Source: three-view drawing plus pictorial views. Frame: mm from the lowest corner of the part. A direction names the side the tool comes from. Give positions to 0.01 mm unless a question says otherwise; leave off trailing zeros. Loops run counter-clockwise (first coordinate to the right, second up) from the corner with the lowest first, then second, coordinate; pieces in that order, holes last. Notation, with made-up numbers: (-25.75, 68) -> (20.25, 68) arc R38 ccw to (20.25, 106) -> close; hole circle Ø7 at (18, 7). An arc over 180 degrees is marked (long way). Answer as a JSON object with one key per item and string values. Group by question number.
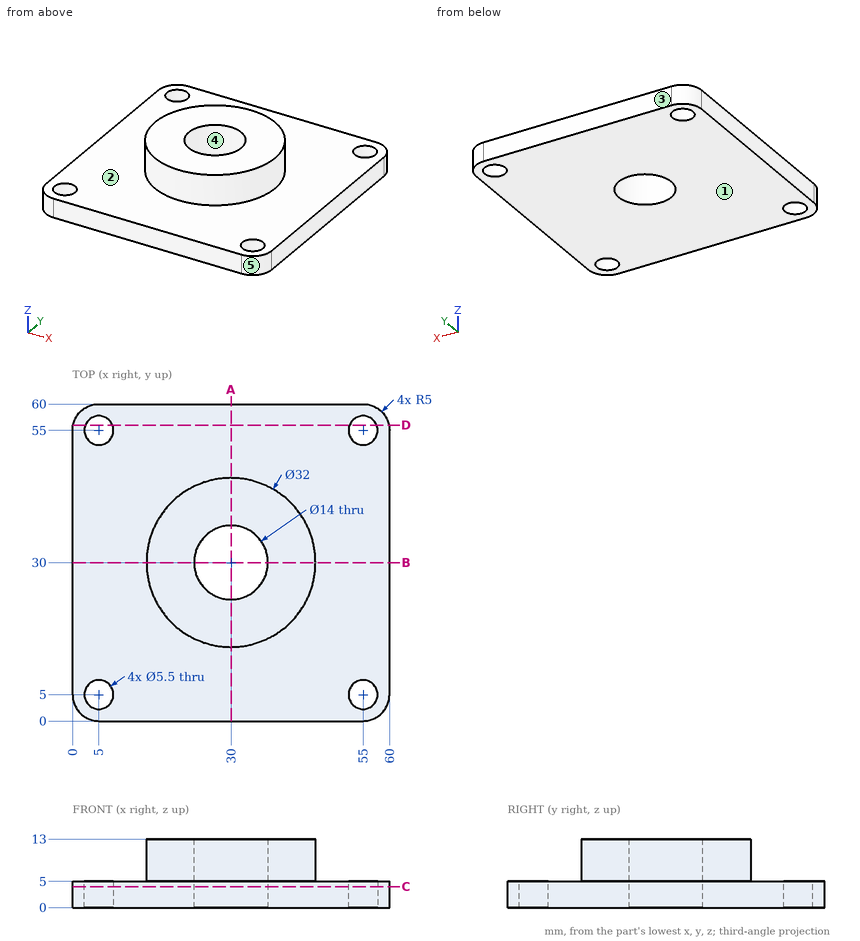
Q1. Pin query (flat end, axial travel): pin 1 Ø6 at (x, z) = (19, 10) entering from +Y; pin 2 Ø5 at (x, y) = (5, 5) entering from -Z; pin 3 Ø1 at (x, z) = (25, 9.5) entering from -Y; pin 4 Ø12 at (x, y) = (52.5, 45.5) entering from +Z. Return the tip coordinate at first contact, or that it passes through.
Q2. Section D-D on y = 56. Return the cut outline in (x, z), then the cut area to 3 significant figures.
Q3. Section C-C on z = 4. Return the cut outline in (x, y), then the cut area to 3 significant figures.
Q4. Section A-A on x = 30. Return the cut outline in (y, z).
Q5. Pull-direction query (Y, two-part tool) for the marked faces 3, 4 and 5; classes: +Y half, -Y half, draft (parallel to the pull), parting line (faces both ways), or undercut.
Q6. Ray query, probe 1 along Y at (x, z) = (5, 1.55); probe 2 along X at (y, z) = (57.5, 4.5); probe 3 along Z at (x, y) = (51.5, 14.5). Return the intervals inside material, ascending.
Q7. Set-up query: the marked faces 1 and 2. Return all of +Z, -Z, +X, -X, +Y, -Y with unobstructed straight access to the full face (end or side cutting, diameter ignored); none if empty.
Numbers:
{
 "1": {"pin 1": "stops at y = 43.86", "pin 2": "passes through", "pin 3": "stops at y = 14.65", "pin 4": "stops at z = 5"},
 "2": {"outline": "(0.1, 0) -> (2.44, 0) -> (2.44, 5) -> (0.1, 5) -> close; (7.56, 0) -> (52.44, 0) -> (52.44, 5) -> (7.56, 5) -> close; (57.56, 0) -> (59.9, 0) -> (59.9, 5) -> (57.56, 5) -> close", "area": "248 mm²"},
 "3": {"outline": "(0, 5) arc R5 ccw to (5, 0) -> (55, 0) arc R5 ccw to (60, 5) -> (60, 55) arc R5 ccw to (55, 60) -> (5, 60) arc R5 ccw to (0, 55) -> close; hole circle Ø5.5 at (5, 5); hole circle Ø5.5 at (5, 55); hole circle Ø14 at (30, 30); hole circle Ø5.5 at (55, 5); hole circle Ø5.5 at (55, 55)", "area": "3,330 mm²"},
 "4": {"outline": "(0, 0) -> (23, 0) -> (23, 13) -> (14, 13) -> (14, 5) -> (0, 5) -> close; (37, 0) -> (60, 0) -> (60, 5) -> (46, 5) -> (46, 13) -> (37, 13) -> close"},
 "5": {"face 3": "+Y half", "face 4": "undercut", "face 5": "-Y half"},
 "6": {"probe 1": "y = 0 to 2.25, 7.75 to 52.25, 57.75 to 60", "probe 2": "x = 0.67 to 3.85, 6.15 to 53.85, 56.15 to 59.33", "probe 3": "z = 0 to 5"},
 "7": {"face 1": "-Z, +X, -X, +Y, -Y", "face 2": "+Z"}
}
